Can you work these out from the model? Positions are in its coordinate system, mm. Face numbers are marked on the shaded views. A direction names the side the tool comes from. Coordinates: 2 decimals unless noted, no trailing zeros. Loops run counter-clockwise (first coordinate to the right, second up) from the corner with the lowest first, then second, coordinate; pieces in that order, holes last. Notation, with made-up numbers: (32.5, 0) - (55.5, 0) arc R25 ccw to (55.5, 28) - close; hole circle Ø1 at (40, -21). An arc over 180 degrees is marked (long way). Put each result on its own line as item: value. Start each with the question number.
from build123d import *

# Parameters (mm, degrees)
CROQUIS1_R              = 17.5
SALIENTE_EXTRUIR1_DEPTH = 11
CROQUIS4_R              = 2
CORTAR_EXTRUIR2_DEPTH   = 28.083205128
CROQUIS6_R              = 2
CORTAR_EXTRUIR3_DEPTH   = 4
SALIENTE_EXTRUIR3_DEPTH = 2
SALIENTE_EXTRUIR4_START = -11
SALIENTE_EXTRUIR4_DEPTH = 11


# Read off the part's stored shape, not the designer's step: Saliente-Extruir3
with BuildPart() as part:
    # Croquis1 → Saliente-Extruir1 (new body)
    with BuildSketch(Plane(origin=(0, 0, 0), x_dir=(1, 0, 0), z_dir=(0, 1, 0))):
        with Locations(Location((0, 0, 0), (0, 0, 270))):
            Circle(CROQUIS1_R)
        with BuildLine():
            ThreePointArc((11.15, 0), (-6.401269405, -9.129416739), (-3.8, 10.482485392))
            Line((-3.8, 10.482485392), (-3.8, 13.15))
            ThreePointArc((-3.8, 13.15), (-3.507106781, 13.857106781), (-2.8, 14.15))
            Line((-2.8, 14.15), (2.8, 14.15))
            ThreePointArc((2.8, 14.15), (3.507106781, 13.857106781), (3.8, 13.15))
            Line((3.8, 13.15), (3.8, 10.482485392))
            ThreePointArc((3.8, 10.482485392), (9.129416739, 6.401269405), (11.15, 0))
        make_face(mode=Mode.SUBTRACT)
    extrude(amount=SALIENTE_EXTRUIR1_DEPTH)

    # Croquis4 → Cortar-Extruir2 (cut, through all)
    with BuildSketch(Plane(origin=(0, 11, 0), x_dir=(1, 0, 0), z_dir=(0, 1, 0))):
        with Locations(Location((-12.557368355, 7.25, 0), (0, 0, 270))):
            Circle(CROQUIS4_R)
        with Locations(Location((12.557368355, 7.25, 0), (0, 0, 270))):
            Circle(CROQUIS4_R)
        with Locations(Location((0, -14.5, 0), (0, 0, 270))):
            Circle(CROQUIS4_R)
    extrude(amount=-CORTAR_EXTRUIR2_DEPTH, mode=Mode.SUBTRACT)

    # Croquis6 → Cortar-Extruir3 (cut)
    with BuildSketch(Plane(origin=(0, 0, 0), x_dir=(-1, 0, 0), z_dir=(0, -1, 0))):
        with Locations(Location((14.325, 0, 0), (0, 0, 90))):
            Circle(CROQUIS6_R)
        with Locations(Location((-14.325, 0, 0), (0, 0, 270))):
            Circle(CROQUIS6_R)
    extrude(amount=-CORTAR_EXTRUIR3_DEPTH, mode=Mode.SUBTRACT)

    # Saliente-Extruir3 outline → Saliente-Extruir3 (add)
    with BuildSketch(Plane(origin=(0, 0, 0), x_dir=(-1, 0, 0), z_dir=(0, -1, 0))):
        with BuildLine():
            ThreePointArc((-10.348912986, 4.15), (-10.00884214, 4.913815118), (-9.612491872, 5.65))
            Line((-9.612491872, 5.65), (-11.357368355, 5.65))
            ThreePointArc((-11.357368355, 5.65), (-12.557368355, 5.25), (-13.757368355, 5.65))
            Line((-13.757368355, 5.65), (-16.562834902, 5.65))
            ThreePointArc((-16.562834902, 5.65), (-16.798572699, 4.904890956), (-17.000808804, 4.15))
            Line((-17.000808804, 4.15), (-10.348912986, 4.15))
        make_face()
        with BuildLine():
            ThreePointArc((-9.612491873, -5.65), (-10.00884214, -4.913815118), (-10.348912986, -4.15))
            Line((-10.348912986, -4.15), (-17.000808804, -4.15))
            ThreePointArc((-17.000808804, -4.15), (-16.798572699, -4.904890956), (-16.562834902, -5.65))
            Line((-16.562834902, -5.65), (-9.612491873, -5.65))
        make_face()
        with BuildLine():
            ThreePointArc((10.348912986, -4.15), (10.00884214, -4.913815118), (9.612491873, -5.65))
            Line((9.612491873, -5.65), (16.562834902, -5.65))
            ThreePointArc((16.562834902, -5.65), (16.798572699, -4.904890956), (17.000808804, -4.15))
            Line((17.000808804, -4.15), (10.348912986, -4.15))
        make_face()
        with BuildLine():
            ThreePointArc((17.000808804, 4.15), (16.798572699, 4.904890956), (16.562834902, 5.65))
            Line((16.562834902, 5.65), (13.757368355, 5.65))
            ThreePointArc((13.757368355, 5.65), (12.557368355, 5.25), (11.357368355, 5.65))
            Line((11.357368355, 5.65), (9.612491872, 5.65))
            ThreePointArc((9.612491872, 5.65), (10.00884214, 4.913815118), (10.348912986, 4.15))
            Line((10.348912986, 4.15), (17.000808804, 4.15))
        make_face()
    extrude(amount=SALIENTE_EXTRUIR3_DEPTH)

    # Croquis11 → Saliente-Extruir4 (add)
    with BuildSketch(Plane(origin=(0, 11, 0), x_dir=(1, 0, 0), z_dir=(0, 1, 0)).offset(SALIENTE_EXTRUIR4_START)):
        with BuildLine():
            Line((-3.8, 10.376054163), (-3.8, 10.482485392))
            ThreePointArc((-3.8, 10.482485392), (-6.401269405, -9.129416739), (11.15, 0))
            ThreePointArc((11.15, 0), (9.129416739, 6.401269405), (3.8, 10.482485392))
            Line((3.8, 10.482485392), (3.8, 10.376054163))
            ThreePointArc((3.8, 10.376054163), (9.057938507, 6.329000711), (11.05, 0))
            ThreePointArc((11.05, 0), (-6.329000711, -9.057938507), (-3.8, 10.376054163))
        make_face()
    extrude(amount=SALIENTE_EXTRUIR4_DEPTH)


solid = part.part
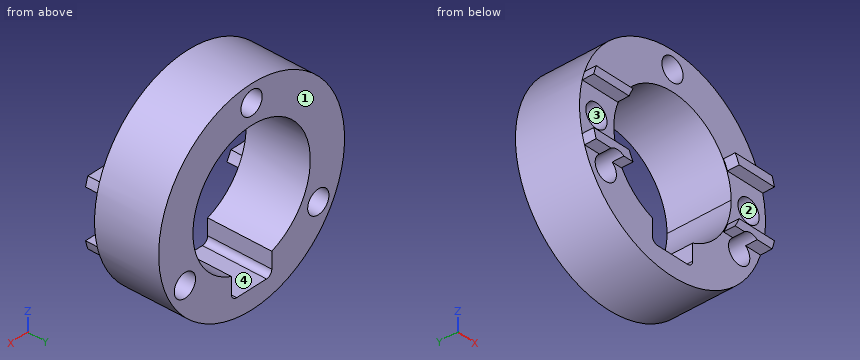
Q1. On a 3-axis mill with a long thin cutter (end or side, diameter ignored), from which of +Z, -Z, +X, -X, +Y, -Y can I reach the whole of each face in a straight line? I mean the marked faces 3 and 4. Say none if no direction works.
Q2. I want a section at D-D on z = 14.5. List the corners of the cut face in (x, y) for me.
Q3. Please list where these lines run through material, in increasing order: line 1 along X through (y, z) = (2, 0) (3 decimals); line 2 along X through (y, z) = (0.5, 1.5); line 3 along X through (y, z) = (3.25, -11). Write a range as [from, to].
Q4. We'd pull the mould along Z, two halves only. Please class the marked faces 1 and 2: released by +Z, released by -Z, zero draft, split by the parting line, or undercut.
Q5. Will these pins go through, and if not, where does the flat tip stop? pin 1 (1.6 mm diameter, centred on x = -12, y = -0.5, fed in from +Z); pin 2 (0.8 mm diameter, centred on y = 5.5, z = -12.5, fed in from +X); pin 3 (2 mm diameter, centred on x = 12, y = -0.5, fed in from +Z).
Q6. I want a section at C-C on x = 9. List the corners of the cut face in (y, z) for me.
Q7. I want a section at B-B on y = 7.25. List the corners of the cut face in (x, z) for me, and give its area (3 significant figures).
Q8. I want a section at A-A on x = 0. List the corners of the cut face in (y, z) for me.
Calculated:
1. face 3: -Y
1. face 4: +Y, -Y
2. outline: (-9.8, 0) - (-2, 0) - (-2, 11) - (-9.8, 11) - close; (2, 0) - (9.8, 0) - (9.8, 11) - (2, 11) - close
3. line 1: [-17.5, -16.325], [-12.325, -11.05], [11.05, 12.325], [16.325, 17.5]
3. line 2: [-17.44, -15.65], [-13, -10.95], [10.95, 13], [15.65, 17.44]
3. line 3: [-13.61, -3.8], [3.8, 13.61]
4. face 1: zero draft
4. face 2: undercut
5. pin 1: z = 13.3
5. pin 2: x = 12.64
5. pin 3: z = 13.5
6. outline: (0, -15.01) - (11, -15.01) - (11, -6.41) - (0, -6.41) - close; (0, 6.41) - (11, 6.41) - (11, 15.01) - (0, 15.01) - close
7. outline: circle Ø35 at (0, 0); hole circle Ø4 at (-12.56, -7.25); hole (-3.8, -13.15) arc R1 ccw to (-2.8, -14.15) - (2.8, -14.15) arc R1 ccw to (3.8, -13.15) - (3.8, -10.38) arc R11.05 ccw (long way) to (-3.8, -10.38) - close; hole circle Ø4 at (0, 14.5); hole circle Ø4 at (12.56, -7.25)
7. area: 516 mm2
8. outline: (0, -17.5) - (11, -17.5) - (11, -14.15) - (0, -14.15) - close; (0, 11.05) - (11, 11.05) - (11, 12.5) - (0, 12.5) - close; (0, 16.5) - (11, 16.5) - (11, 17.5) - (0, 17.5) - close
